from build123d import *

# Parameters (mm, degrees)
F0_W     = 95
F0_H     = 65
F0_W_2   = 93
F0_H_2   = 63
F1_DEPTH = 12
F2_DEPTH = 2
F3_W     = 1
F3_H     = 3
F4_DEPTH = 1.5
F5_W     = 1
F5_H     = 3
F6_DEPTH = 14
F7_W     = 95
F7_H     = 65
F7_W_2   = 93
F7_H_2   = 63
F8_DEPTH = 2


with BuildPart() as f1:
    # F0 (on Top) → F1 (new body)
    with BuildSketch(Plane.XY):
        Rectangle(F0_W, F0_H)
        Rectangle(F0_W_2, F0_H_2, mode=Mode.SUBTRACT)
    extrude(amount=F1_DEPTH)

    # F0 (on Top) → F2 (join)
    with BuildSketch(Plane.XY):
        Rectangle(F0_W_2, F0_H_2)
    extrude(amount=F2_DEPTH)

    # F3 (on face) → F4 (join)
    with BuildSketch(Plane.XY.offset(12)):
        Polygon((47.5, 32.5), (-47.5, 32.5), (-47.5, 25.5), (-46.5, 25.5), (-46.5, 31.5), (46.5, 31.5), (46.5, -31.5), (-46.5, -31.5), (-46.5, -7.5), (-47.5, -7.5), (-47.5, -32.5), (47.5, -32.5), align=None)
        with Locations((-47, 9)):
            Rectangle(F3_W, F3_H)
    extrude(amount=F4_DEPTH)

    # F5 (on face) → F6 (join)
    with BuildSketch(Plane.XY.offset(13.5)):
        Polygon((47.5, -32.5), (47.5, 32.5), (-47.5, 32.5), (-47.5, 25.5), (-46.5, 25.5), (-46.5, 31.5), (46.5, 31.5), (46.5, -31.5), (-46.5, -31.5), (-46.5, -26.5), (-47.5, -26.5), (-47.5, -32.5), align=None)
        with Locations((-47, -9)):
            Rectangle(F5_W, F5_H)
        with Locations((-47, 9)):
            Rectangle(F5_W, F5_H)
    extrude(amount=F6_DEPTH)

    # F7 (on face) → F8 (join)
    with BuildSketch(Plane.XY.offset(27.5)):
        Rectangle(F7_W, F7_H)
        Rectangle(F7_W_2, F7_H_2, mode=Mode.SUBTRACT)
    extrude(amount=F8_DEPTH)


solid = f1.part
Verification items for the finished model (mm, model axes). A direction names the side the tool comes from. Round coordinates to 2 decimals unless told otherwise and drop trailing zeros. Loops run counter-clockwise (first coordinate to the right, second up) from the corner with the lowest first, then second, coordinate; pieces in that order, holes last. Notation, with made-up numbers: (4.5, 31) - (33.5, 31) arc R22 ccw to (33.5, 52) - close; hole circle Ø3 at (41.25, 64). An arc over 180 degrees is marked (long way). Answer in a Markdown table with one row per item. Add a question column.
Q1. Section check A-A on z = 22. Enter the section's corners in (x, y).
Q2. Section check B-B on y = 12.5. Enter the section's corners in (x, z), plus the area to 4 significant figures.
Q3. Release check for a two-part mould opening along X. For faces 1 (the face through (-1, 32.5, 15)), 2 (the face through (-1, 0, 2)), 3 (the face through (-47.5, 0, 11)) record: pulls with the +X half, pulls with the -X half, needs draft (parallel to the pull), parting line crosses it, or undercut.
Q4. Gauge pin test, flat end, axial feed: pin 1 (19 mm diameter, centred on x = 19, y = -6.5, fed in from +Z). Record the tip position at first contact, or that the pin passes through.
Q5. Section check D-D on x = -39.5. Enter the section's corners in (y, z), plus the area to 3 significant figures.
Q6. Tool access check on faces 4 (the face through (-1, 31.5, 16)), 5 (the face through (-1, -32.5, 15)). Record the directions out of +Z, -Z, +X, -X, +Y, -Y that give a thin tool (end or side, any length) a straight path to the whole face; none if there is none.
Q7. Section check C-C on z = 4. Enter the section's corners in (x, y), plus the area to 3 significant figures.
Q8. Material ranges on line 1 (X direction, y = 9, z = 22.75); line 2 (Y direction, x = 6.5, z = 26.75); line 3 (X direction, y = -15, z = 23.5), recorded low to high.
Found:
| question | item | result |
|---|---|---|
| 1 | outline | (-47.5, -32.5) - (47.5, -32.5) - (47.5, 32.5) - (-47.5, 32.5) - (-47.5, 25.5) - (-46.5, 25.5) - (-46.5, 31.5) - (46.5, 31.5) - (46.5, -31.5) - (-46.5, -31.5) - (-46.5, -26.5) - (-47.5, -26.5) - close; (-47.5, -10.5) - (-46.5, -10.5) - (-46.5, -7.5) - (-47.5, -7.5) - close; (-47.5, 7.5) - (-46.5, 7.5) - (-46.5, 10.5) - (-47.5, 10.5) - close |
| 2 | outline | (-47.5, 0) - (47.5, 0) - (47.5, 29.5) - (46.5, 29.5) - (46.5, 2) - (-46.5, 2) - (-46.5, 12) - (-47.5, 12) - close; (-47.5, 27.5) - (-46.5, 27.5) - (-46.5, 29.5) - (-47.5, 29.5) - close |
| 2 | area | 229.5 mm² |
| 3 | face 1 | needs draft |
| 3 | face 2 | undercut |
| 3 | face 3 | pulls with the -X half |
| 4 | pin 1 | stops at z = 2 |
| 5 | outline | (-32.5, 0) - (32.5, 0) - (32.5, 29.5) - (31.5, 29.5) - (31.5, 2) - (-31.5, 2) - (-31.5, 29.5) - (-32.5, 29.5) - close |
| 5 | area | 185 mm² |
| 6 | face 4 | +Z |
| 6 | face 5 | +Z, -Z, +X, -X, -Y |
| 7 | outline | (-47.5, -32.5) - (47.5, -32.5) - (47.5, 32.5) - (-47.5, 32.5) - close; hole (-46.5, -31.5) - (46.5, -31.5) - (46.5, 31.5) - (-46.5, 31.5) - close |
| 7 | area | 316 mm² |
| 8 | line 1 | x = -47.5 to -46.5, 46.5 to 47.5 |
| 8 | line 2 | y = -32.5 to -31.5, 31.5 to 32.5 |
| 8 | line 3 | x = 46.5 to 47.5 |
